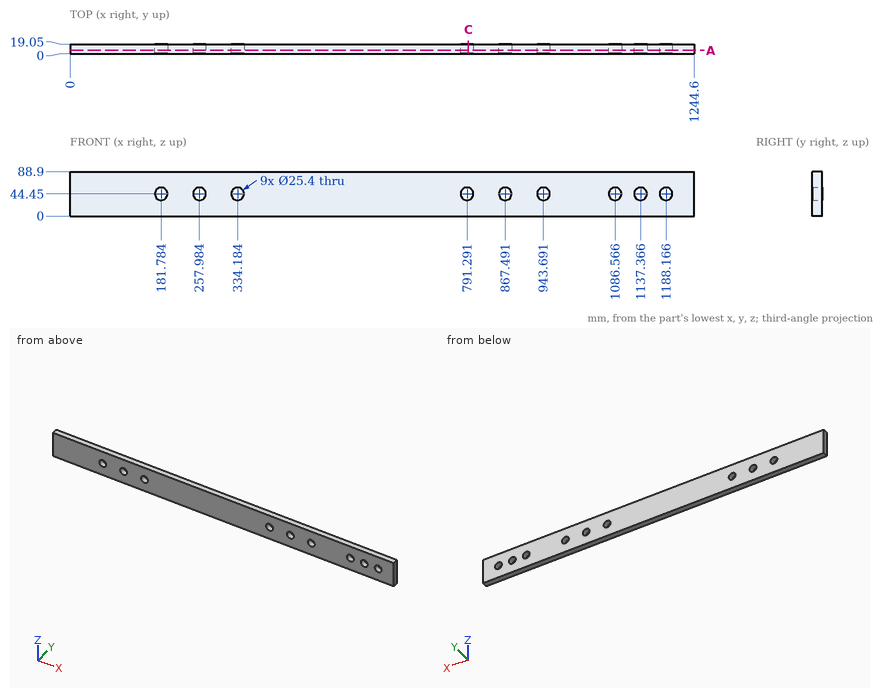
Print and shaded views of the part. All mm, measured from the part's lowest x, y and z. Coordinates: 2 decimals unless noted, no trailing zeros. Loops run counter-clockwise (first coordinate to the right, second up) from the corner with the lowest first, then second, coordinate; pieces in that order, holes last. Notation, with made-up numbers: (14, -20.75) -> (55, -20.75) arc R19 ccw to (55, -4.75) -> close; hole circle Ø7 at (-38, -4.5). An arc over 180 degrees is marked (long way). Use one line per item in the form item = value. Start each with the question number.
(1) Probe probe 1 along Z at (x, y) = (870, 9.5); probe 2 along Z at (x, y) = (877.5, 17.75) (1 decimal). List the from-to ranges inside material, lowest first. Write a range as from..to.
(2) Cut at A-A on y = 6.25. Give the number of separate pieces and of enclosed holes in the cut face, and give its area (3 significant figures).
(3) Cut at C-C on x = 794. Give the cut face in (y, z), and give its area (3 significant figures).
Values:
q1.probe_1 = 0..32, 56.9..88.9
q1.probe_2 = 0..36.6, 52.3..88.9
q2.separate_pieces = 1
q2.enclosed_holes = 9
q2.area = 106,000 mm2
q3.outline = (0, 0) -> (19.05, 0) -> (19.05, 32.04) -> (0, 32.04) -> close; (0, 56.86) -> (19.05, 56.86) -> (19.05, 88.9) -> (0, 88.9) -> close
q3.area = 1,220 mm2
